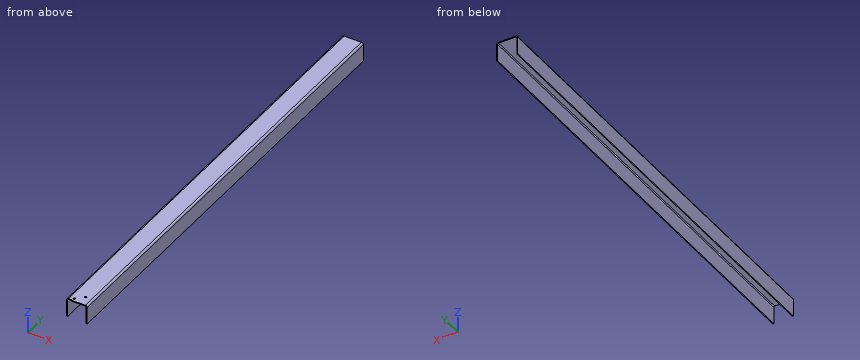
```python
from build123d import *

# Parameters (mm, degrees)
F1_DEPTH = 1996
F3_W     = 4
F3_H     = 87
F4_DEPTH = 21.409
F6_R     = 4.5
F5_R     = 4.5
F7_DEPTH = 4


with BuildPart() as f1:
    # F0 (on Front) → F1 (new body)
    with BuildSketch(Plane.XZ):
        with BuildLine():
            Line((-46.25, 34), (-46.25, -42))
            Line((-46.25, -42), (-42.25, -42))
            Line((-42.25, -42), (-42.25, 34))
            ThreePointArc((-42.25, 34), (-41.078427, 36.828427), (-38.25, 38))
            Line((-38.25, 38), (38.25, 38))
            ThreePointArc((38.25, 38), (41.078427, 36.828427), (42.25, 34))
            Line((42.25, 34), (42.25, -42))
            Line((42.25, -42), (46.25, -42))
            Line((46.25, -42), (46.25, 34))
            ThreePointArc((46.25, 34), (43.906854, 39.656854), (38.25, 42))
            Line((38.25, 42), (-38.25, 42))
            ThreePointArc((-38.25, 42), (-43.906854, 39.656854), (-46.25, 34))
        make_face()
    extrude(amount=-F1_DEPTH)

    # F3 (on face) → F4 (cut)
    with BuildSketch(Plane(origin=(-46.25, 0, 0), x_dir=(0, -1, 0), z_dir=(-1, 0, 0))):
        with Locations((-2, 0.370724)):
            Rectangle(F3_W, F3_H)
    extrude(amount=-F4_DEPTH, mode=Mode.SUBTRACT)

    # F6 (on face) + F5 (on face) → F7 (cut)
    with BuildSketch(Plane(origin=(0, 0, 38), x_dir=(1, 0, 0), z_dir=(0, 0, -1))):
        with Locations((12.063, -45.5)):
            Circle(F6_R)
    with BuildSketch(Plane(origin=(0, 0, 38), x_dir=(1, 0, 0), z_dir=(0, 0, -1))):
        with Locations((-18.92, -14.5)):
            Circle(F5_R)
    extrude(amount=-F7_DEPTH, mode=Mode.SUBTRACT)


solid = f1.part
```
Geometry check sheet. Reference: the model listing, model coordinates, mm. Give positions to 0.01 mm unless a question says otherwise; leave off trailing zeros. Write each loop counter-clockwise with the first axis right and the second up, starting at its lowest first coordinate (ties: lowest second). Pieces come first, ordered by that corner, then holes.
1) Section check A-A, the plane z = -16.5. Record the boundary of the cut face in (x, y), and give its area (3 significant figures).
2) Material ranges on L1, parallel to X at y = 431, z = 10; L2, parallel to Y at x = -18, z = 39; L3, parallel to Z at x = 23.5, y = 1488, recorded low to high.
3) Section check B-B, the plane y = 600.5. Record the boundary of the cut face in (x, z), and give its area (3 significant figures).
4) Gauge pin test, flat ends, axial feed: pin 1 (12 mm diameter, centred on x = -5, z = 27, fed in from -Y); pin 2 (4.5 mm diameter, centred on y = 2, z = 39.5, fed in from -X); pin 3 (2 mm diameter, centred on x = 5.5, y = 1746.5, fed in from -Z); pin 4 (10.5 mm diameter, centred on x = -39, z = -9, fed in from -Y). Record the tip position at first contact, or that the pin passes through.
Computed:
1. outline: (-46.25, 4) - (-42.25, 4) - (-42.25, 1996) - (-46.25, 1996) - close; (42.25, 0) - (46.25, 0) - (46.25, 1996) - (42.25, 1996) - close
1. area: 16,000 mm2
2. L1: x = -46.25 to -42.25, 42.25 to 46.25
2. L2: y = 0 to 10.1, 18.9 to 1996
2. L3: z = 38 to 42
3. outline: (-46.25, -42) - (-42.25, -42) - (-42.25, 34) arc R4 cw to (-38.25, 38) - (38.25, 38) arc R4 cw to (42.25, 34) - (42.25, -42) - (46.25, -42) - (46.25, 34) arc R8 ccw to (38.25, 42) - (-38.25, 42) arc R8 ccw to (-46.25, 34) - close
3. area: 989 mm2
4. pin 1: passes through
4. pin 2: stops at x = -44.89
4. pin 3: stops at z = 38
4. pin 4: stops at y = 4
